from build123d import *

# Parameters (mm, degrees)
SKETCH2_W           = 6
SKETCH2_H           = 30
BOSS_EXTRUDE1_DEPTH = 30
SKETCH4_R           = 2.775
CUT_EXTRUDE2_DEPTH  = 30
SKETCH5_R           = 1.7
CUT_EXTRUDE3_DEPTH  = 39


with BuildPart() as part:
    # Sketch2 → Boss-Extrude1 (new body)
    with BuildSketch(Plane(origin=(0, 0, 0), x_dir=(0, 0, -1), z_dir=(1, 0, 0))):
        Rectangle(SKETCH2_W, SKETCH2_H)
        Polygon((-3, 19), (-3, 15), (3, 15), (33, 15), (33, 19), align=None)
        Polygon((3, -15), (-3, -15), (-3, -19), (33, -19), (33, -15), align=None)
    extrude(amount=BOSS_EXTRUDE1_DEPTH)

    # Sketch4 → Cut-Extrude2 (cut)
    with BuildSketch(Plane.XY.offset(3)):
        with Locations((15, 0)):
            Circle(SKETCH4_R)
    extrude(amount=-CUT_EXTRUDE2_DEPTH, mode=Mode.SUBTRACT)

    # Sketch5 → Cut-Extrude3 (cut, through all)
    with BuildSketch(Plane.XZ.offset(19)):
        with Locations((15, -18)):
            Circle(SKETCH5_R)
    extrude(amount=-CUT_EXTRUDE3_DEPTH, mode=Mode.SUBTRACT)


solid = part.part
Geometry: final body of the model. Coordinates: model frame, mm. A direction names the side the tool comes from. Round coordinates to 2 decimals unless told otherwise and drop trailing zeros. Write each loop counter-clockwise with the first axis right and the second up, starting at its lowest first coordinate (ties: lowest second). Pieces come first, ordered by that corner, then holes. Notation, with made-up numbers: M 43.25,11 L 54.25,11 A29 cw 54.25,31 Z; hole C -24,-36.5 d3. An arc over 180 degrees is marked long. Write item = value, one per line.
Item 1: Access query for faces 5 (the face through (30, 0.3, -2.7)), 6 (the face through (15, -4, -3)). Directions: +Z, -Z, +X, -X, +Y, -Y. A direction counts if a zero-diameter tool reaches every point of the face in a straight line with its end or side. Return the directions, or none.
Findings:
face_5 = +Z, -Z, +X, +Y, -Y
face_6 = -Z, +X, -X
Item 2: Section query D-D on x = 15. Return loops of the section in (y, z) (3 decimals).
Findings:
outline = M -19,-33 L -15,-33 L -15,-19.7 L -19,-19.7 Z; M -19,-16.3 L -15,-16.3 L -15,-3 L -2.775,-3 L -2.775,3 L -19,3 Z; M 2.775,-3 L 15,-3 L 15,-16.3 L 19,-16.3 L 19,3 L 2.775,3 Z; M 15,-33 L 19,-33 L 19,-19.7 L 15,-19.7 Z
Item 3: Section query B-B on y = 0. Return loops of the section in (x, z) (3 decimals).
Findings:
outline = M 0,-3 L 12.225,-3 L 12.225,3 L 0,3 Z; M 17.775,-3 L 30,-3 L 30,3 L 17.775,3 Z
Item 4: Pin query (flat end, axial travel): P1, Ø1, axis at y = 13.5, z = -4.5, coming from the +X side; P2, Ø9, axis at x = 19.5, y = -7, coming from the -Z side. Return the tip coordinate at first contact, or that it passes through.
Findings:
P1 = through
P2 = -3
Item 5: Section query C-C on z = -18. Return loops of the section in (x, y), then the cut area to 3 significant figures.
Findings:
outline = M 0,-19 L 13.3,-19 L 13.3,-15 L 0,-15 Z; M 0,15 L 13.3,15 L 13.3,19 L 0,19 Z; M 16.7,-19 L 30,-19 L 30,-15 L 16.7,-15 Z; M 16.7,15 L 30,15 L 30,19 L 16.7,19 Z
area = 213 mm^2
Item 6: Material intervals for line 1 along Y through (x, z) = (11.75, -11); line 2 along Z through (x, y) = (15, -16.6); line 3 along Z through (x, y) = (24.25, -1), sorted ascending. Write a range as [from, to].
Findings:
line_1 = [-19, -15], [15, 19]
line_2 = [-33, -19.7], [-16.3, 3]
line_3 = [-3, 3]
Item 7: Section query A-A on z = -13. Return loops of the section in (x, y).
Findings:
outline = M 0,-19 L 30,-19 L 30,-15 L 0,-15 Z; M 0,15 L 30,15 L 30,19 L 0,19 Z
Item 8: Pull-direction query (X, two-part tool) for faces 1 (the face through (0, 0.3, -2.7)), 2 (the face through (15, -19, -15)), 3 (the face through (15.914, -17.028, -16.567)), 4 (the face through (12.228, 0.122, 0.042)); classes: pulls with the +X half, pulls with the -X half, needs draft (parallel to the pull), parting line crosses it, or undercut.
Findings:
face_1 = pulls with the -X half
face_2 = needs draft
face_3 = undercut
face_4 = undercut
